Input: part model. Units: mm. Frame: model coordinates. A direction names the side the tool comes from. Round coordinates to 2 decimals unless told otherwise and drop trailing zeros. Loops run counter-clockwise (first coordinate to the right, second up) from the corner with the lowest first, then second, coordinate; pieces in that order, holes last. Notation, with made-up numbers: (-37, -7.75) -> (13, -7.75) arc R30 ccw to (13, 31.25) -> close; hole circle Ø6 at (60.25, 83.25). An arc over 180 degrees is marked (long way). Answer as a JSON object with one key per item and string values.
```python
from build123d import *

# Parameters (mm, degrees)
F9_DEPTH = 5
F10_R    = 2


with BuildPart() as f2:
    # F2: sweep along a path in F1
    with BuildLine(Plane.YZ) as f2_path:
        Line((0, 0), (0, 45))
        ThreePointArc((0, 45), (5.8578643763, 59.1421356237), (20, 65))
        Line((20, 65), (110, 65))
    # F0 (on Top) → F2 (sweep)
    with BuildSketch(Plane.XY):
        with BuildLine():
            ThreePointArc((14, 0), (-0.5, 10.478936224), (-15, 0))
            Line((-15, 0), (-11.6882403352, 0))
            ThreePointArc((-11.6882403352, 0), (-0.5, 7.3789365762), (10.6882403352, 0))
            Line((10.6882403352, 0), (14, 0))
        make_face()
    sweep(path=f2_path.line)

    # F6: sweep along a path in F4
    with BuildLine(Plane.XZ) as f6_path:
        Line((0, 0), (0, -25.4587277886))
        ThreePointArc((0, -25.4587277886), (5.8578643763, -39.6008634124), (20, -45.4587277886))
        Line((20, -45.4587277886), (30, -45.4587277886))
    # F0 (on Top) → F6 (sweep)
    with BuildSketch(Plane.XY):
        with BuildLine():
            ThreePointArc((14, 0), (-0.5, 10.478936224), (-15, 0))
            Line((-15, 0), (-11.6882403352, 0))
            ThreePointArc((-11.6882403352, 0), (-0.5, 7.3789365762), (10.6882403352, 0))
            Line((10.6882403352, 0), (14, 0))
        make_face()
    sweep(path=f6_path.line)

    # F6_face (on face) → F7 section 0
    with BuildSketch(Plane(origin=(30, 5.8470332672, -45.9587277886), x_dir=(0, 1, 0), z_dir=(1, 0, 0))):
        with BuildLine():
            Line((-5.8470332672, -11.1882403352), (-5.8470332672, -14.5))
            ThreePointArc((-5.8470332672, -14.5), (4.6319029568, 0), (-5.8470332672, 14.5))
            Line((-5.8470332672, 14.5), (-5.8470332672, 11.1882403352))
            ThreePointArc((-5.8470332672, 11.1882403352), (1.5319033089, 0), (-5.8470332672, -11.1882403352))
        make_face()
    # F5 (on offset) → F7 section 1
    with BuildSketch(Plane.YZ.offset(79.5)):
        with BuildLine():
            Line((-10.8751536487, -37.9657093932), (-13.9526978979, -37.2235111379))
            ThreePointArc((-13.9526978979, -37.2235111379), (1.4814826902, -58.6311098034), (12.4912671201, -34.6460340717))
            Line((12.4912671201, -34.6460340717), (10.1624930815, -36.7332008739))
            ThreePointArc((10.1624930815, -36.7332008739), (0.7118567894, -55.5823045887), (-10.8751536487, -37.9657093932))
        make_face()
    loft()

    # F5 (on offset) + F8 (on face) → F9 (join)
    with BuildSketch(Plane.YZ.offset(79.5)):
        with BuildLine():
            Line((-10.8751536487, -37.9657093932), (-13.9526978979, -37.2235111379))
            ThreePointArc((-13.9526978979, -37.2235111379), (1.4814826902, -58.6311098034), (12.4912671201, -34.6460340717))
            Line((12.4912671201, -34.6460340717), (10.1624930815, -36.7332008739))
            ThreePointArc((10.1624930815, -36.7332008739), (0.7118567894, -55.5823045887), (-10.8751536487, -37.9657093932))
        make_face()
    with BuildSketch(Plane.YZ.offset(79.5)):
        with BuildLine():
            Line((12.4912671201, -34.6460340717), (10.1624930815, -36.7332008739))
            ThreePointArc((10.1624930815, -36.7332008739), (0.7118567894, -55.5823045887), (-10.8751536487, -37.9657093932))
            Line((-10.8751536487, -37.9657093932), (-13.9526978979, -37.2235111379))
            ThreePointArc((-13.9526978979, -37.2235111379), (1.4814826902, -58.6311098034), (12.4912671201, -34.6460340717))
        make_face()
        with BuildLine():
            ThreePointArc((-10.8751536487, -37.9657093932), (0.7118567894, -55.5823045887), (10.1624930815, -36.7332008739))
            Line((10.1624930815, -36.7332008739), (12.4912671201, -34.6460340717))
            Line((12.4912671201, -34.6460340717), (-13.9526978979, -37.2235111379))
            Line((-13.9526978979, -37.2235111379), (-10.8751536487, -37.9657093932))
        make_face()
    extrude(amount=F9_DEPTH)

    # F10
    f10_edges = [f2.edges().sort_by_distance(p)[0] for p in [
        (84.5, 1.481483, -58.63111),
        (79.5, 1.481483, -58.63111),
    ]]
    fillet(f10_edges, radius=F10_R)


solid = f2.part
```
1) Section B-B, the plane y = 27. Output: boundary loops of the cut face in (x, z), plus the area to 3 significant figures.
Output:
{"outline": "(-15, 65) arc R15.27 ccw to (14, 65) -> (10.69, 65) arc R12.17 cw to (-11.69, 65) -> close", "area": "103 mm^2"}
2) Contact query for flat-ended pins moving along their axis: P1, Ø6, axis at x = 17.5, y = 47.5, coming from the +Z side (3 decimals); P2, Ø13.5, axis at x = 8.5, z = -17, coming from the -Y side; P3, Ø5, axis at x = 67, y = 1.5, coming from the -Z side. Output: stop coordinate, or through.
Output:
{"P1": "passes through", "P2": "stops at y = 0", "P3": "stops at z = -56.42"}
3) Ray query, probe 1 along X at (y, z) = (-1, -37.5); probe 2 along Z at (x, y) = (-7, 43); probe 3 along Y at (x, z) = (5.5, 2). Return the intervals inside material, ascending.
Output:
{"probe 1": "x = 79.5 to 84.5", "probe 2": "z = 55.97 to 59.5", "probe 3": "y = 5.8 to 9.25"}
4) Section A-A, the plane z = 38. Output: boundary loops of the cut face in (x, y).
Output:
{"outline": "(-15, 0) -> (-11.69, 0) arc R12.17 cw to (10.69, 0) -> (14, 0) arc R15.27 ccw to start"}
5) Reachability of faces 4 (the face through (-0.699, 7.377, 9.277)), 5 (the face through (-13, 0, -16)), 6 (the face through (-0.232, 65.63, 54.523)) from +Z, -Z, +X, -X, +Y, -Y: full face, straight path, thin tool, end or side. Return the list, or none.
Output:
{"face 4": "+Z, -Y", "face 5": "+Z, -Z, -X, -Y", "face 6": "-Z, +Y"}
6) Draft query along Z for faces 1 (the face through (-0.768, 10.477, 9.277)), 2 (the face through (13, 0, 2)), 3 (the face through (-0.301, 65.63, 57.623)). Return one class per face: +Z half, -Z half, draft (parallel to the pull), parting line (faces both ways), or undercut.
Output:
{"face 1": "undercut", "face 2": "draft", "face 3": "+Z half"}
